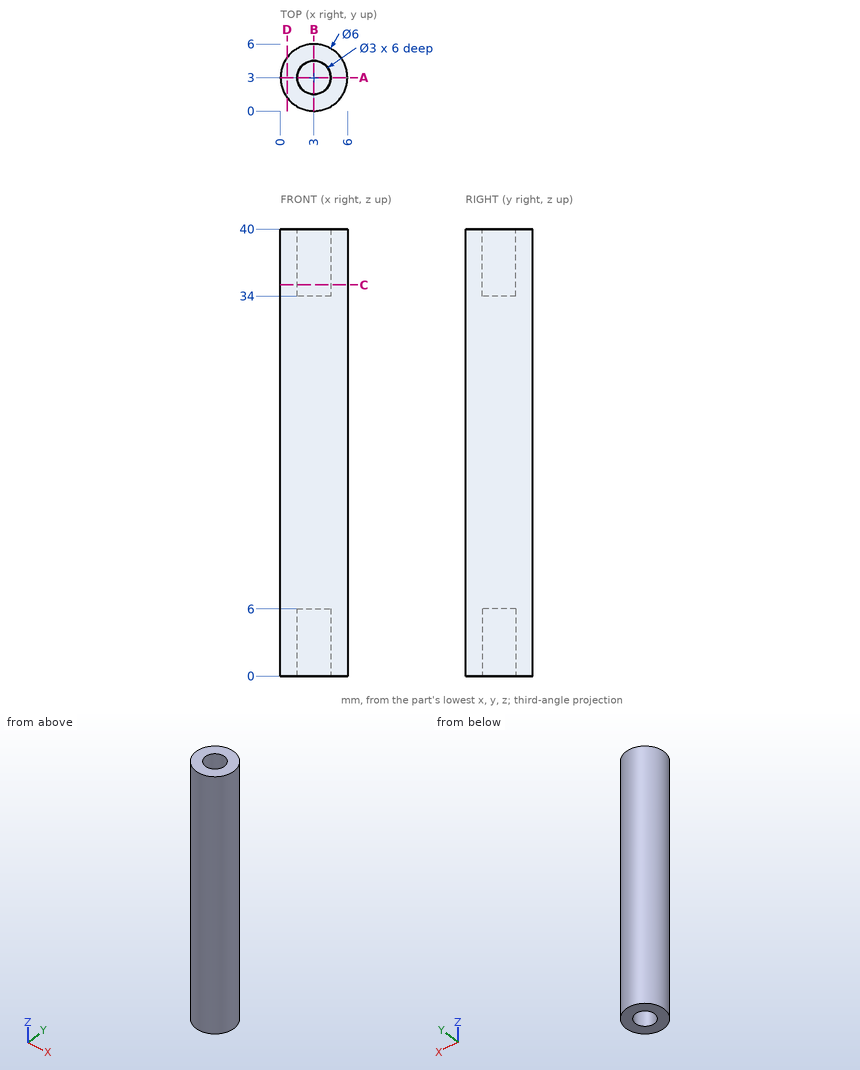
Job drawing, mm, ordinate dimensions from the low corner. One solid piece. Give positions to 0.01 mm unless a question says otherwise; leave off trailing zeros. Order: outer loops, then holes, each group sorted by start corner. A loop starts at its lowest first (then second) coordinate and runs counter-clockwise, first axis right, second up. Notation, with made-up numbers: (-30.75, 16.25) - (15.25, 16.25) arc R31 cw to (15.25, 54.25) - close; hole circle Ø2 at (49.25, 85.25). An arc over 180 degrees is marked (long way). Answer in a Markdown table with one row per item.
1. Saw through at A-A, the plane y = 3. Give the cut face in (x, z).
Data:
| item | result |
|---|---|
| outline | (0, 0) - (1.5, 0) - (1.5, 6) - (4.5, 6) - (4.5, 0) - (6, 0) - (6, 40) - (4.5, 40) - (4.5, 34) - (1.5, 34) - (1.5, 40) - (0, 40) - close |
2. Saw through at D-D, the plane x = 0.6. Give the cut face in (y, z), plus the area to 3 significant figures.
Data:
| item | result |
|---|---|
| outline | (1.2, 0) - (4.8, 0) - (4.8, 40) - (1.2, 40) - close |
| area | 144 mm² |
3. Saw through at C-C, the plane z = 35. Give the cut face in (x, y), plus the area to 3 significant figures.
Data:
| item | result |
|---|---|
| outline | circle Ø6 at (3, 3); hole circle Ø3 at (3, 3) |
| area | 21.2 mm² |
4. Probe probe 1 along Y at (x, z) = (3, 3.4); probe 2 along Z at (x, y) = (3.95, 2.3); probe 3 along X at (y, z) = (2.9, 11.5). List the from-to ranges inside material, lowest first. Write a range as [from, to].
Data:
| item | result |
|---|---|
| probe 1 | y = [0, 1.5], [4.5, 6] |
| probe 2 | z = [6, 34] |
| probe 3 | x = [0, 6] |
5. Flat gauge pins, fed straight in: pin 1 (2.5 mm diameter, centred on x = 3, y = 3, fed in from -Z); pin 2 (1 mm diameter, centred on x = 1, z = 32, fed in from +Y); pin 3 (1.5 mm diameter, centred on x = 2.5, y = 3.5, fed in from +Z). Where does each tip first touch, or does it go through?
Data:
| item | result |
|---|---|
| pin 1 | stops at z = 6 |
| pin 2 | stops at y = 5.6 |
| pin 3 | stops at z = 34 |
